from build123d import *

# Parameters (mm, degrees)
PAD_DEPTH       = 1
SKETCH012_R     = 9
POCKET_DEPTH    = 1.001
POCKET001_DEPTH = 1.001
PAD003_DEPTH    = 10


with BuildPart() as part:
    # Sketch007 → Pad (new body)
    with BuildSketch(Plane.XY):
        with BuildLine():
            Line((13.5, 15.5), (-13.5, 15.5))
            ThreePointArc((-15.469616, 17.152704), (-14.785575, 15.967911), (-13.5, 15.5))
            Line((-15.469616, 17.152704), (-16.153704, 21.03236))
            ThreePointArc((-16.153704, 21.03236), (-17.281843, 22.891476), (-19.369594, 23.5))
            Line((-19.369594, 23.5), (-26.098892, 22.911263))
            ThreePointArc((-26.098892, 22.911263), (-32.808142, 21.113525), (-38.497913, 17.129504))
            Line((-40.313708, 15.313708), (-38.497913, 17.129504))
            ThreePointArc((-40.313708, 15.313708), (-43.782073, 10.122935), (-45, 4))
            Line((-45, 4), (-45, 0))
            Line((-45, 0), (30.5, 0))
            Line((30.5, 0), (30.5, 10.677124))
            ThreePointArc((30.75, 11.338562), (30.564586, 11.030678), (30.5, 10.677124))
            ThreePointArc((30.75, 11.338562), (30.935414, 11.646447), (31, 12))
            Line((31, 17.015221), (31, 12))
            ThreePointArc((31, 17.015221), (29.702361, 19.964331), (26.651377, 21))
            Line((18.276649, 20.267306), (26.651377, 21))
            ThreePointArc((18.276649, 20.267306), (16.511345, 19.490554), (15.583693, 17.799667))
            Line((15.583693, 17.799667), (15.469616, 17.152704))
            ThreePointArc((13.5, 15.5), (14.785575, 15.967911), (15.469616, 17.152704))
        make_face()
        with BuildLine():
            Line((-20, 13), (-17, 13))
            ThreePointArc((-17, 13), (-16.25, 13.75), (-17, 14.5))
            Line((-20, 14.5), (-17, 14.5))
            ThreePointArc((-20, 14.5), (-20.75, 13.75), (-20, 13))
        make_face(mode=Mode.SUBTRACT)
        with BuildLine():
            Line((-1.5, 13), (1.5, 13))
            ThreePointArc((1.5, 13), (2.25, 13.75), (1.5, 14.5))
            Line((-1.5, 14.5), (1.5, 14.5))
            ThreePointArc((-1.5, 14.5), (-2.25, 13.75), (-1.5, 13))
        make_face(mode=Mode.SUBTRACT)
        with BuildLine():
            Line((17, 13), (20, 13))
            ThreePointArc((20, 13), (20.75, 13.75), (20, 14.5))
            Line((17, 14.5), (20, 14.5))
            ThreePointArc((17, 14.5), (16.25, 13.75), (17, 13))
        make_face(mode=Mode.SUBTRACT)
    pad = extrude(amount=PAD_DEPTH)

    # Mirrored: Pad across Sketch007 H_Axis
    add(pad.mirror(Plane.ZX))

    # Sketch012 (on Face5 of Mirrored) → Pocket (cut, through all)
    with BuildSketch(Plane.XY.offset(1)):
        Circle(SKETCH012_R)
    extrude(amount=-POCKET_DEPTH, mode=Mode.SUBTRACT)

    # Sketch008 → Pocket001 (cut, through all)
    with BuildSketch(Plane.XY):
        with BuildLine():
            Line((-41.5, 2.732233), (-41.5, -2.732233))
            ThreePointArc((-41.5, -2.732233), (-39.956709, -5.041932), (-37.232233, -4.5))
            Line((-35.792893, -3.06066), (-37.232233, -4.5))
            ThreePointArc((-35.792893, -3.06066), (-35.57612, -2.736237), (-35.5, -2.353553))
            Line((-35.5, 2.353553), (-35.5, -2.353553))
            ThreePointArc((-35.5, 2.353553), (-35.57612, 2.736237), (-35.792893, 3.06066))
            Line((-37.232233, 4.5), (-35.792893, 3.06066))
            ThreePointArc((-37.232233, 4.5), (-39.956709, 5.041932), (-41.5, 2.732233))
        make_face()
    extrude(amount=POCKET001_DEPTH, mode=Mode.SUBTRACT)

    # Sketch → Pad003 (join)
    with BuildSketch(Plane.XY):
        Polygon((-40.913498, 8.863434), (-210.841839, -238.383837), (-215.131018, -235.380521), align=None)
        Polygon((-36.380804, 5.7482), (-208.460287, -240.006771), (-204.145063, -242.972542), align=None)
        Polygon((-25.08387, 19.530617), (-321.799927, 63.875129), (-322.528654, 58.689966), align=None)
    pad003 = extrude(amount=PAD003_DEPTH)

    # Mirrored001: Pad003 across Sketch H_Axis
    add(pad003.mirror(Plane.ZX))


solid = part.part
Here's how the part is built. I have some questions about the finished solid (model axes, mm). A direction names the side the tool comes from. Coordinates: 2 decimals unless noted, no trailing zeros. Order: outer loops, then holes, each group sorted by start corner. A loop starts at its lowest first (then second) coordinate and runs counter-clockwise, first axis right, second up. Notation, with made-up numbers: M 89.5,-39.5 L 141.5,-39.5 A17 ccw 141.5,-23.5 Z; hole C 28,58 d1. An arc over 180 degrees is marked long. Answer as CSV lines item,"result". Start each with the question number.
1. We'd pull the mould along Y, two halves only. Please class faces 4 (the flat face through (-40.626, -21.853, 4.93)), 5 (the flat face through (-50.315, 14.152, 4.93)), 6 (the flat face through (-133, 35, 0)), 7 (the cylindrical face through (-1.172, 8.923, 0.507)): released by +Y, released by -Y, zero draft, split by the parting line, or undercut.
2. On a 3-axis mill with a long thin cutter (end or side, diameter ignored), from which of +Z, -Z, +X, -X, +Y, -Y can I reach the whole of each face in a straight line? I mean faces 1 (the flat face through (-141.35, -131.94, 4.93)), 2 (the flat face through (-56.195, -12.56, 4.93)), 3 (the flat face through (-131.41, 135.14, 4.93)). Say none if no direction works.
3. I want a section at D-D, the plane y = -109. Write out the boundary of the cut face in (x, z).
4. I want a section at B-B, the plane x = -119.5. Write out the boundary of the cut face in (y, z), and give its area (3 significant figures).
5. I need wall thicknesses on line 1 (Y direction, x = 0, z = 0.7); line 2 (Y direction, x = -168, z = 1.75); line 3 (Y direction, x = -63.5, z = 3.25). Which ranges of each line are inside material? Lowest first, please. Write a range as [from, to].
6. For pin 1 (0.8 mm diameter, centred on x = -18.5, z = 0.5, fed in from -Y); pin 2 (1.1 mm diameter, centred on x = -6.5, z = 0.5, fed in from -Y); pin 3 (1.5 mm diameter, centred on y = -157.5, z = 9, fed in from -X); pin 4 (23.5 mm diameter, centred on x = 0, y = 0, fed in from -Z), each with a flat end and sliding along its axis, tell me the tip position at first contact or that it passes through.
7. I want a section at A-A, the plane y = 161. Write out the boundary of the cut face in (x, z).
8. I want a section at C-C, the plane z = 7. Count the separate pieces of the cut face and the enclosed holes in it, and give its area (3 significant figures).
Recorded:
1,face 4,"released by -Y"
1,face 5,"undercut"
1,face 6,"zero draft"
1,face 7,"undercut"
2,face 1,"+Z, -Z"
2,face 2,"+Z, -Z, -X"
2,face 3,"+Z, -Z, +X, +Y"
3,outline,"M -124.98,0 L -121.92,0 L -121.92,10 L -124.98,10 Z; M -116.73,0 L -113.78,0 L -113.78,10 L -116.73,10 Z"
4,outline,"M -117.48,0 L -112.96,0 L -112.96,10 L -117.48,10 Z; M -105.48,0 L -101.31,0 L -101.31,10 L -105.48,10 Z; M -33.64,0 L -31.96,0 L -31.96,10 L -33.64,10 Z; M 31.96,0 L 33.64,0 L 33.64,10 L 31.96,10 Z; M 101.31,0 L 105.48,0 L 105.48,10 L 101.31,10 Z; M 112.96,0 L 117.48,0 L 117.48,10 L 112.96,10 Z"
4,area,"207 mm2"
5,line 1,"y = [-15.5, -14.5], [-13, -9], [9, 13], [14.5, 15.5]"
5,line 2,"y = [-189.39, -182.22], [-176.05, -169.31], [-40.89, -38.35], [38.35, 40.89], [169.31, 176.05], [182.22, 189.39]"
5,line 3,"y = [-34.46, -32.98], [-25.27, -24.59], [-24, -22.8], [22.8, 24], [24.59, 25.27], [32.98, 34.46]"
6,pin 1,"stops at y = -23.5"
6,pin 2,"stops at y = -15.5"
6,pin 3,"stops at x = -160.11"
6,pin 4,"stops at z = 0"
7,outline,"M -162.08,0 L -157.66,0 L -157.66,10 L -162.08,10 Z; M -153.14,0 L -148.85,0 L -148.85,10 L -153.14,10 Z"
8,separate pieces,"1"
8,enclosed holes,"3"
8,area,"4,710 mm2"
